Verification items for the finished model (mm, model axes). A direction names the side the tool comes from. Give positions to 0.01 mm unless a question says otherwise; leave off trailing zeros. Write each loop counter-clockwise with the first axis right and the second up, starting at its lowest first coordinate (ties: lowest second). Pieces come first, ordered by that corner, then holes. Notation, with made-up numbers: M 43.25,82.5 L 61.25,82.5 A12 cw 61.25,105.5 Z; hole C -30.5,32 d5. An arc over 180 degrees is marked long. Answer as a JSON object with one key per item and string values.
```python
from build123d import *

# Parameters (mm, degrees)
SKETCH1_W           = 40
SKETCH1_H           = 40
BOSS_EXTRUDE1_DEPTH = 10
FILLET1_R           = 3.5
SKETCH2_R           = 2
CUT_EXTRUDE1_DEPTH  = 11
CUT_EXTRUDE2_DEPTH  = 11
CIRPATTERN1_COUNT   = 12
SKETCH6_R           = 17.5
CUT_EXTRUDE3_DEPTH  = 1


with BuildPart() as part:
    # Sketch1 → Boss-Extrude1 (new body)
    with BuildSketch(Plane.XY):
        Rectangle(SKETCH1_W, SKETCH1_H)
    extrude(amount=BOSS_EXTRUDE1_DEPTH)

    # Fillet1
    fillet1_edges = [part.edges().sort_by_distance(p)[0] for p in [
        (20, -20, 5),
        (-20, -20, 5),
        (-20, 20, 5),
        (20, 20, 5),
    ]]
    fillet(fillet1_edges, radius=FILLET1_R)

    # Sketch2 → Cut-Extrude1 (cut, through all)
    with BuildSketch(Plane.XY.offset(10)):
        with Locations((16.5, -16.5)):
            Circle(SKETCH2_R)
        with Locations((16.5, 16.5)):
            Circle(SKETCH2_R)
        with Locations((-16.5, 16.5)):
            Circle(SKETCH2_R)
        with Locations((-16.5, -16.5)):
            Circle(SKETCH2_R)
    extrude(amount=-CUT_EXTRUDE1_DEPTH, mode=Mode.SUBTRACT)

    # Sketch5 → Cut-Extrude2 (cut, through all)
    with BuildSketch(Plane.XY.offset(10)):
        with BuildLine():
            Line((17.350285074, 2.284208364), (9.914448614, 1.305261922))
            ThreePointArc((9.914448614, 1.305261922), (9.978589232, 0.654031292), (10, 0))
            ThreePointArc((10, 0), (9.978589232, -0.654031292), (9.914448614, -1.305261922))
            Line((9.914448614, -1.305261922), (17.350285074, -2.284208364))
            ThreePointArc((17.350285074, -2.284208364), (17.462531157, -1.144554762), (17.5, 0))
            ThreePointArc((17.5, 0), (17.462531157, 1.144554762), (17.350285074, 2.284208364))
        make_face()
    cut_extrude2 = extrude(amount=-CUT_EXTRUDE2_DEPTH, mode=Mode.SUBTRACT)

    # CirPattern1: Cut-Extrude2 ×12 about axis
    cirpattern1_axis = Axis((0, 0, 0), (0, 0, 1))
    for i in range(1, CIRPATTERN1_COUNT):
        add(cut_extrude2.rotate(cirpattern1_axis, i * 360 / CIRPATTERN1_COUNT), mode=Mode.SUBTRACT)

    # Sketch6 → Cut-Extrude3 (cut)
    with BuildSketch(Plane.XY.offset(10)):
        Circle(SKETCH6_R)
    extrude(amount=-CUT_EXTRUDE3_DEPTH, mode=Mode.SUBTRACT)


solid = part.part
```
1) Thickness scan on L1, parallel to X at y = 17, z = 1.5; L2, parallel to X at y = -16, z = 1.75; L3, parallel to Y at x = -13, z = 5.75. Record the ranges inside material, lowest first.
Completed:
{"L1": "x = -19.96 to -18.44, -14.56 to -2.24, 2.24 to 14.56, 18.44 to 19.96", "L2": "x = -20 to -18.44, -14.56 to -7.09, -6.63 to -2.11, 2.11 to 6.63, 7.09 to 14.56, 18.44 to 20", "L3": "y = -20 to -9.98, -5.38 to -1.71, 1.71 to 5.38, 9.98 to 20"}
2) Section check D-D on z = 2.5. Count the separate pieces of the cut face and the enclosed holes in it, and give its area (3 significant figures).
Completed:
{"separate pieces": "1", "enclosed holes": "16", "area": "1,220 mm2"}
3) Section check C-C on x = 13. Record the boundary of the cut face in (y, z), and give its area (3 significant figures).
Completed:
{"outline": "M -20,0 L -9.98,0 L -9.98,9 L -11.72,9 L -11.72,10 L -20,10 Z; M -5.38,0 L -1.71,0 L -1.71,9 L -5.38,9 Z; M 1.71,0 L 5.38,0 L 5.38,9 L 1.71,9 Z; M 9.98,0 L 20,0 L 20,10 L 11.72,10 L 11.72,9 L 9.98,9 Z", "area": "263 mm2"}
4) Access from +Z, -Z, +X, -X, +Y, -Y to the whole of each face (thin tool, end or side, straight path). Record for faces 1 (the face through (0, 20, 5)), 2 (the face through (-13.58, 1.788, 4.563)).
Completed:
{"face 1": "+Z, -Z, +X, -X, +Y", "face 2": "+Z, -Z"}
5) Section check B-B on y = -11.5. Record the boundary of the cut face in (x, z), and give its area (3 significant figures).
Completed:
{"outline": "M -20,0 L -8.82,0 L -8.82,9 L -13.19,9 L -13.19,10 L -20,10 Z; M -4.76,0 L -1.51,0 L -1.51,9 L -4.76,9 Z; M 1.51,0 L 4.76,0 L 4.76,9 L 1.51,9 Z; M 8.82,0 L 20,0 L 20,10 L 13.19,10 L 13.19,9 L 8.82,9 Z", "area": "273 mm2"}
6) Go/stop test with a flat-tipped pin: pin 1 (17.5 mm diameter, centred on x = -0.5, y = 2, fed in from +Z). Record where the tip stops, or that it passes through.
Completed:
{"pin 1": "stops at z = 9"}
7) Section check A-A on x = -5.5. Record the boundary of the cut face in (y, z), and give its area (3 significant figures).
Completed:
{"outline": "M -20,0 L -13.28,0 L -13.28,9 L -16.61,9 L -16.61,10 L -20,10 Z; M -8.35,0 L 8.35,0 L 8.35,9 L -8.35,9 Z; M 13.28,0 L 20,0 L 20,10 L 16.61,10 L 16.61,9 L 13.28,9 Z", "area": "278 mm2"}
